Model file for the job. Use its own axes, mm. A direction names the side the tool comes from. Give positions to 0.01 mm unless a question says otherwise; leave off trailing zeros. Order: outer loops, then holes, each group sorted by start corner. A loop starts at its lowest first (then second) coordinate and runs counter-clockwise, first axis right, second up. Notation, with made-up numbers: (-25, 67.25) -> (17, 67.25) arc R16 cw to (17, 76.25) -> close; hole circle Ø6 at (77.5, 42). An arc over 180 degrees is marked (long way). Answer in a Markdown table with one row per item. Add a question column.
from build123d import *

# Parameters (mm, degrees)
F1_DEPTH  = 25
F2_DEPTH  = 1
F3_DEPTH  = 1
F4_W      = 6
F4_H      = 11
F4_H_2    = 1
F5_DEPTH  = 25
F6_R      = 3
F6_R_2    = 1.625
F7_DEPTH  = 7
F8_DEPTH  = 2
F9_DEPTH  = 1
F10_R     = 0.75
F11_DEPTH = 0.5
F12_R     = 0.75


with BuildPart() as f1:
    # F0 (on Top) → F1 (new body)
    with BuildSketch(Plane.XY):
        with BuildLine():
            Line((0, 9), (0, 0))
            Line((0, 0), (12, 0))
            Line((12, 0), (12, 9))
            Line((12, 9), (8.2360679775, 9))
            ThreePointArc((8.2360679775, 9), (6, 4), (3.7639320225, 9))
            Line((3.7639320225, 9), (0, 9))
        make_face()
    extrude(amount=F1_DEPTH)

    # F2 (cut): a face of the model
    f2_faces = [f1.faces().sort_by_distance(p)[0] for p in [
        (0, 4.5, 12.5),
    ]]
    extrude(f2_faces, amount=-F2_DEPTH, mode=Mode.SUBTRACT)

    # F3 (cut): a face of the model
    f3_faces = [f1.faces().sort_by_distance(p)[0] for p in [
        (12, 4.5, 12.5),
    ]]
    extrude(f3_faces, amount=-F3_DEPTH, mode=Mode.SUBTRACT)

    # F4 (on face) → F5 (cut)
    with BuildSketch(Plane.YZ.offset(11)):
        with Locations((6, 14.5)):
            Rectangle(F4_W, F4_H)
        with Locations((6, 0.5)):
            Rectangle(F4_W, F4_H_2)
    extrude(amount=-F5_DEPTH, mode=Mode.SUBTRACT)

    # F6 (on face) → F7 (cut)
    with BuildSketch(Plane.XZ):
        with Locations((6, 5)):
            Circle(F6_R)
        with Locations((6, 5)):
            Circle(F6_R_2, mode=Mode.SUBTRACT)
        with Locations((6, 5)):
            Circle(F6_R_2)
    extrude(amount=-F7_DEPTH, mode=Mode.SUBTRACT)

    # F6 (on face) → F8 (join)
    with BuildSketch(Plane.XZ):
        with Locations((6, 5)):
            Circle(F6_R)
        with Locations((6, 5)):
            Circle(F6_R_2, mode=Mode.SUBTRACT)
    extrude(amount=-F8_DEPTH)

    # F9 (cut): a face of the model
    f9_faces = [f1.faces().sort_by_distance(p)[0] for p in [
        (6, 1.5, 0),
    ]]
    extrude(f9_faces, amount=-F9_DEPTH, mode=Mode.SUBTRACT)

    # F10
    f10_edges = [f1.edges().sort_by_distance(p)[0] for p in [
        (8.236068, 9, 5),
        (3.763932, 9, 5),
        (3.763932, 9, 22.5),
        (8.236068, 9, 22.5),
    ]]
    fillet(f10_edges, radius=F10_R)

    # F11 (cut): a face of the model
    f11_faces = [f1.faces().sort_by_distance(p)[0] for p in [
        (6, 3, 14.5),
    ]]
    extrude(f11_faces, amount=-F11_DEPTH, mode=Mode.SUBTRACT)

    # F12
    f12_edges = [f1.edges().sort_by_distance(p)[0] for p in [
        (11, 2.5, 14.5),
        (1, 2.5, 14.5),
    ]]
    fillet(f12_edges, radius=F12_R)


solid = f1.part
Item 1: Saw through at B-B on z = 3.75. List the corners of the cut face in (x, y), plus the area to 3 significant figures.
Item 2: Which spindle directions (+Z, -Z, +X, -X, +Y, -Y) get a long thin tool onto all of the face, cutting with end or side? Do faces 1 (the cylindrical face through (3, 4, 5)), 2 (the flat face through (10, 9, 5)), 3 (the cylindrical face through (3.083, 8.675, 5.056)). Say none if no direction does.
Item 3: Saw through at D-D on z = 16.5. List the corners of the cut face in (x, y), plus the area to 3 significant figures.
Item 4: Pin check, flat tips, straight feed: pin 1 Ø4 at (x, z) = (7, 12) entering from +Y; pin 2 Ø3 at (x, z) = (7.5, 5) entering from +Y; pin 3 Ø3 at (y, z) = (3.5, 17) entering from +X. Stop position of each tip, or through.
Item 5: Wall check: line 1 (X direction, y = 7, z = 23.35); line 2 (Z direction, x = 1.75, y = 3); line 3 (Z direction, x = 6, y = 0.8) (3 decimals). Give the ranges that are in metal, low to high.
Item 6: Two-plate mould, pull along Z, no slides. Class faces 4 (the cylindrical face through (4.802, 0.986, 6.098)), 5 (the flat face through (6, 2.5, 14)), 6 (the flat face through (5.9, 3.6, 1)), 7 (the cylindrical face through (3.07, 8.69, 22.54)): pulls with the +Z half, pulls with the -Z half, needs draft (parallel to the pull), parting line crosses it, or undercut.
Item 7: Saw through at C-C on y = 7.5. List the corners of the cut face in (x, z), plus the area to 3 significant figures.
Item 8: Saw through at A-A on x = 6. List the corners of the cut face in (y, z) (3 decimals), plus the area to 3 significant figures.
Evaluation:
| question | item | result |
|---|---|---|
| 1 | outline | (1, 0) -> (4.96, 0) -> (4.96, 2) -> (3.27, 2) -> (3.27, 5.75) arc R3 cw to (3.17, 8) arc R0.75 ccw to (2.46, 9) -> (1, 9) -> close; (7.04, 0) -> (11, 0) -> (11, 9) -> (9.54, 9) arc R0.75 ccw to (8.83, 8) arc R3 cw to (8.73, 5.75) -> (8.73, 2) -> (7.04, 2) -> close |
| 1 | area | 46.4 mm2 |
| 2 | face 1 | none |
| 2 | face 2 | +Z, -Z, +X, -X, +Y |
| 2 | face 3 | +Z, -Z |
| 3 | outline | (1, 0) -> (11, 0) -> (11, 1.75) arc R0.75 ccw to (10.25, 2.5) -> (1.75, 2.5) arc R0.75 ccw to (1, 1.75) -> close |
| 3 | area | 24.8 mm2 |
| 4 | pin 1 | stops at y = 2.5 |
| 4 | pin 2 | stops at y = 8.78 |
| 4 | pin 3 | stops at x = 10.96 |
| 5 | line 1 | x = 1 to 3, 9 to 11 |
| 5 | line 2 | z = 1 to 9, 20 to 25 |
| 5 | line 3 | z = 1 to 3.375, 6.625 to 25 |
| 6 | face 4 | undercut |
| 6 | face 5 | undercut |
| 6 | face 6 | pulls with the -Z half |
| 6 | face 7 | needs draft |
| 7 | outline | (1, 1) -> (3.04, 1) -> (3.04, 9) -> (1, 9) -> close; (1, 20) -> (3.04, 20) -> (3.04, 25) -> (1, 25) -> close; (8.96, 1) -> (11, 1) -> (11, 9) -> (8.96, 9) -> close; (8.96, 20) -> (11, 20) -> (11, 25) -> (8.96, 25) -> close |
| 7 | area | 53.1 mm2 |
| 8 | outline | (0, 1) -> (4, 1) -> (4, 2) -> (2, 2) -> (2, 3.375) -> (0, 3.375) -> close; (0, 6.625) -> (2, 6.625) -> (2, 8) -> (4, 8) -> (4, 9) -> (2.5, 9) -> (2.5, 20) -> (4, 20) -> (4, 25) -> (0, 25) -> close |
| 8 | area | 61.0 mm2 |
